Work out the finished part from the listing and answer in its coordinate system (mm). A direction names the side the tool comes from. Coordinates: 2 decimals unless noted, no trailing zeros. Order: outer loops, then holes, each group sorted by start corner. A loop starts at its lowest first (then second) coordinate and runs counter-clockwise, first axis right, second up.
1. Find the intervals of material crossed by probe 1 along X at (y, z) = (1.25, -3.5); probe 2 along Z at (x, y) = (-1.5, 2.75), in increasing order.
2. A tool of negligible diameter and unlimited length cuts with its end or side. For faces 1 (the flat face through (0, 7, 3)), 2 (the flat face through (0, 3, 7)), 3 (the flat face through (-17, 3, 2)), 4 (the flat face through (0, 4, 0)), 5 (the cylindrical face through (17.701, 3.47, 1.994)), from which of +Z, -Z, +X, -X, +Y, -Y can it reach the whole face along a straight path? Write none if from no direction.
3. The part is cut by section A-A, the plane x = -12. Give the vertices of the cut face in (y, z), then the cut area to 3 significant figures.
4. Determine the mould class of faces 6 (the cylindrical face through (30.246, 9.942, 1.994)), 7 (the flat face through (0, 1, -7)), 8 (the flat face through (33.038, 10, 3)) for opening direction Z: +Z half, -Z half, draft (parallel to the pull), parting line (faces both ways), or undercut.
5. The part is cut by section C-C, the plane x = 10. Give the vertices of the cut face in (y, z).
6. The part is cut by section D-D, the plane z = 5.75. Give the vertices of the cut face in (x, y).
7. Flat-ended cylindrical pins translate along their axes: pin 1 Ø3 at (x, z) = (-12, -3.5) entering from +Y; pin 2 Ø3 at (x, z) = (12, -3.5) entering from -Y; pin 3 Ø2.5 at (x, y) = (4.5, 4) entering from -Z; pin 4 Ø5.5 at (x, z) = (2, 4) entering from +Y. Find the tip coordinate at first contact, or state that the pin passes through.
8. The part is cut by section B-B, the plane z = -3.5. Give the vertices of the cut face in (x, y), then the cut area to 3 significant figures.
```python
from build123d import *

# Parameters (mm, degrees)
SKETCH1_W           = 34
SKETCH1_H           = 14
BOSS_EXTRUDE1_DEPTH = 2
SKETCH2_W           = 34
SKETCH2_H           = 7
BOSS_EXTRUDE2_DEPTH = 5
FILLET1_R           = 0.5
CUT_EXTRUDE1_REACH  = 21.053
SKETCH3_R           = 1.25


with BuildPart() as part:
    # Sketch1 → Boss-Extrude1 (new body)
    with BuildSketch(Plane(origin=(0, 0, 0), x_dir=(1, 0, 0), z_dir=(0, 1, 0))):
        Rectangle(SKETCH1_W, SKETCH1_H)
    extrude(amount=BOSS_EXTRUDE1_DEPTH)

    # Sketch2 → Boss-Extrude2 (add)
    with BuildSketch(Plane(origin=(0, 2, 0), x_dir=(1, 0, 0), z_dir=(0, 1, 0))):
        with Locations((0, -3.5)):
            Rectangle(SKETCH2_W, SKETCH2_H)
    extrude(amount=BOSS_EXTRUDE2_DEPTH)

    # Fillet1
    fillet1_edges = [part.edges().sort_by_distance(p)[0] for p in [
        (17, 4.5, 0),
        (-17, 4.5, 0),
        (17, 3.5, 7),
        (-17, 3.5, 7),
        (-17, 1, -7),
        (17, 1, -7),
    ]]
    fillet(fillet1_edges, radius=FILLET1_R)

    # Sketch3 → Cut-Extrude1 (cut, up to next)
    with BuildSketch(Plane(origin=(0, 2, 0), x_dir=(1, 0, 0), z_dir=(0, 1, 0)), mode=Mode.PRIVATE) as cut_extrude1_sk1:
        with Locations(Location((12, 3.5, 0), (0, 0, 270))):
            Circle(SKETCH3_R)
    cut_extrude1_tool1 = extrude(cut_extrude1_sk1.sketch, amount=-CUT_EXTRUDE1_REACH, mode=Mode.PRIVATE) & part.part
    # Sketch3 → Cut-Extrude1 (cut, up to next)
    with BuildSketch(Plane(origin=(0, 2, 0), x_dir=(1, 0, 0), z_dir=(0, 1, 0)), mode=Mode.PRIVATE) as cut_extrude1_sk2:
        with Locations(Location((-12, 3.5, 0), (0, 0, 270))):
            Circle(SKETCH3_R)
    cut_extrude1_tool2 = extrude(cut_extrude1_sk2.sketch, amount=-CUT_EXTRUDE1_REACH, mode=Mode.PRIVATE) & part.part
    add(cut_extrude1_tool1.solids().sort_by_distance((12, 2, -3.5))[0], mode=Mode.SUBTRACT)
    add(cut_extrude1_tool2.solids().sort_by_distance((-12, 2, -3.5))[0], mode=Mode.SUBTRACT)

    # Sweep1: sweep along a path in Sketch5
    with BuildLine(Plane.XY.offset(3.5)) as sweep1_path:
        Line((17, 3.5), (18.382578008, 3.5))
        ThreePointArc((18.382578008, 3.5), (19.635477623, 3.904030935), (20.416306226, 4.963891838))
        ThreePointArc((20.416306226, 4.963891838), (23.087486641, 8.589629512), (27.373601284, 9.971801625))
        Line((27.373601284, 9.971801625), (33.038157501, 9.971801625))
    # Sketch4 → Sweep1 (sweep)
    with BuildSketch(Plane(origin=(17, 0, 0), x_dir=(0, 0, -1), z_dir=(1, 0, 0))):
        with BuildLine():
            ThreePointArc((-3.5, 3.874862619), (-5.006737587, 3.5), (-3.5, 3.125137381))
            ThreePointArc((-3.5, 3.125137381), (-1.993262413, 3.5), (-3.5, 3.874862619))
        make_face()
    sweep(path=sweep1_path.line)


solid = part.part
```
Geometry says:
1. probe 1: x = -17 to -13.25, -10.75 to 10.75, 13.25 to 17
1. probe 2: z = 0 to 7
2. face 1: +Z, -Z, -X, +Y
2. face 2: +Z, +X, -X, +Y, -Y
2. face 3: +Z, -Z, -X, +Y, -Y
2. face 4: -Z, +X, -X, +Y
2. face 5: none
3. outline: (0, -7) - (2, -7) - (2, -4.75) - (0, -4.75) - close; (0, -2.25) - (2, -2.25) - (2, 0) - (7, 0) - (7, 7) - (0, 7) - close
3. area: 58.0 mm2
4. face 6: undercut
4. face 7: -Z half
4. face 8: draft
5. outline: (0, -7) - (2, -7) - (2, 0) - (7, 0) - (7, 7) - (0, 7) - close
6. outline: (-17, 0) - (17, 0) - (17, 7) - (-17, 7) - close
7. pin 1: stops at y = 2
7. pin 2: stops at y = 0
7. pin 3: stops at z = 0
7. pin 4: stops at y = 7
8. outline: (-17, 0) - (-13.25, 0) - (-13.25, 2) - (-17, 2) - close; (-10.75, 0) - (10.75, 0) - (10.75, 2) - (-10.75, 2) - close; (13.25, 0) - (17, 0) - (17, 2) - (13.25, 2) - close
8. area: 58.0 mm2
